Source: CAD feature listing. Evaluate the final solid. Frame: model axes, mm. A direction names the side the tool comes from. Give positions to 0.01 mm unless a question says otherwise; leave off trailing zeros. Order: outer loops, then holes, each group sorted by start corner. A loop starts at its lowest first (then second) coordinate and runs counter-clockwise, first axis right, second up. Notation, with made-up numbers: (84, 9) -> (100, 9) arc R22 cw to (100, 16) -> close; hole circle Ø1 at (87, -12.75). An arc over 180 degrees is marked (long way). Use one line per item in the form item = value. Start each with the question number.
from build123d import *

# Parameters (mm, degrees)
BOSS_EXTRUDE1_DEPTH = 80
SKETCH3_W           = 20
SKETCH3_H           = 40
CUT_EXTRUDE1_DEPTH  = 25
SKETCH4_W           = 55
SKETCH4_H           = 5
CUT_EXTRUDE2_DEPTH  = 40
SKETCH6_W           = 20
SKETCH6_H           = 5
CUT_EXTRUDE3_DEPTH  = 40
SKETCH7_W           = 20
SKETCH7_H           = 10
CUT_EXTRUDE4_DEPTH  = 20
SKETCH8_W           = 10
SKETCH8_H           = 10
BOSS_EXTRUDE2_DEPTH = 20
SKETCH9_W           = 15
SKETCH9_H           = 10
CUT_EXTRUDE5_DEPTH  = 20
SKETCH11_W          = 15
SKETCH11_H          = 5
CUT_EXTRUDE6_DEPTH  = 40


with BuildPart() as part:
    # Sketch1 → Boss-Extrude1 (new body)
    with BuildSketch(Plane(origin=(0, 0, 0), x_dir=(0, 0, -1), z_dir=(1, 0, 0))):
        Polygon((0, 0), (0, -15), (40, -15), (40, 25), (0, 25), (0, 10), (20, 10), (20, 0), align=None)
    extrude(amount=-BOSS_EXTRUDE1_DEPTH)

    # Sketch3 → Cut-Extrude1 (cut)
    with BuildSketch(Plane.XZ.offset(15)):
        with Locations((-40, -20)):
            Rectangle(SKETCH3_W, SKETCH3_H)
    extrude(amount=-CUT_EXTRUDE1_DEPTH, mode=Mode.SUBTRACT)

    # Sketch4 → Cut-Extrude2 (cut)
    with BuildSketch(Plane.XY):
        with Locations((-37.5, 12.5)):
            Rectangle(SKETCH4_W, SKETCH4_H)
    extrude(amount=-CUT_EXTRUDE2_DEPTH, mode=Mode.SUBTRACT)

    # Sketch6 → Cut-Extrude3 (cut)
    with BuildSketch(Plane.XY):
        with Locations((-20, -2.5)):
            Rectangle(SKETCH6_W, SKETCH6_H)
    extrude(amount=-CUT_EXTRUDE3_DEPTH, mode=Mode.SUBTRACT)

    # Sketch7 → Cut-Extrude4 (cut)
    with BuildSketch(Plane.XY.offset(-20)):
        with Locations((-20, 5)):
            Rectangle(SKETCH7_W, SKETCH7_H)
    extrude(amount=-CUT_EXTRUDE4_DEPTH, mode=Mode.SUBTRACT)

    # Sketch8 → Boss-Extrude2 (add)
    with BuildSketch(Plane.XY.offset(-20)):
        with Locations((-5, 5)):
            Rectangle(SKETCH8_W, SKETCH8_H)
    extrude(amount=BOSS_EXTRUDE2_DEPTH)

    # Sketch9 → Cut-Extrude5 (cut)
    with BuildSketch(Plane.XY.offset(-20)):
        with Locations((-57.5, 5)):
            Rectangle(SKETCH9_W, SKETCH9_H)
    extrude(amount=-CUT_EXTRUDE5_DEPTH, mode=Mode.SUBTRACT)

    # Sketch11 → Cut-Extrude6 (cut)
    with BuildSketch(Plane(origin=(0, 0, -40), x_dir=(-1, 0, 0), z_dir=(0, 0, -1))):
        with Locations((57.5, -2.5)):
            Rectangle(SKETCH11_W, SKETCH11_H)
    extrude(amount=-CUT_EXTRUDE6_DEPTH, mode=Mode.SUBTRACT)


solid = part.part
1) Cut plane C-C, the plane x = -53.5. Return the cut outline in (y, z), plus the area to 3 significant figures.
2) Cut plane B-B, the plane y = -4. Return the cut outline in (x, z).
3) Draft query along Y for faces 1 (the face through (-50, -10, -20)), 2 (the face through (-15, -15, -20)), 3 (the face through (-73, 0, -10)), 4 (the face through (-38, 15, -20)). Return one class per face: +Y half, -Y half, draft (parallel to the pull), parting line (faces both ways), or undercut.
4) Reachability of faces 5 (the face through (-80, 5, -24)), 6 (the face through (-72, 10, -10)), 7 (the face through (-20, -5, -20)), 8 (the face through (-30, -10, -20)) from +Z, -Z, +X, -X, +Y, -Y: full face, straight path, thin tool, end or side. Return the list, or none.
5) Cut plane D-D, the plane z = -27. Return the cut outline in (x, y).
6) Cut plane A-A, the plane z = -5. Return the cut outline in (x, y), plus the area to 3 significant figures.
7) Material intervals for probe 1 along X at (y, z) = (4.5, -25); probe 2 along Y at (x, z) = (-24.5, -2.5); probe 3 along X at (y, z) = (-12.5, -30.5), sorted ascending.
8) Pin query (flat end, axial travel): pin 1 (3 mm diameter, centred on x = -37.5, z = -20.5, fed in from -Y); pin 2 (5 mm diameter, centred on x = -71, y = 6.5, fed in from +Z). Return the tip coordinate at first contact, or that it passes through.
Output values:
q1.outline = (-15, -40) -> (-5, -40) -> (-5, 0) -> (-15, 0) -> close; (15, -40) -> (25, -40) -> (25, 0) -> (15, 0) -> close
q1.area = 800 mm^2
q2.outline = (-80, -40) -> (-65, -40) -> (-65, 0) -> (-80, 0) -> close; (-10, -40) -> (0, -40) -> (0, 0) -> (-10, 0) -> close
q3.face_1 = draft
q3.face_2 = -Y half
q3.face_3 = undercut
q3.face_4 = undercut
q4.face_5 = +Z, -Z, -X, +Y, -Y
q4.face_6 = +Z, -X
q4.face_7 = +Z, -Z
q4.face_8 = +Z, -Z, -Y
q5.outline = (-80, -15) -> (-50, -15) -> (-50, -5) -> (-65, -5) -> (-65, 15) -> (-10, 15) -> (-10, -5) -> (-30, -5) -> (-30, -15) -> (0, -15) -> (0, 25) -> (-80, 25) -> close
q6.outline = (-80, -15) -> (-50, -15) -> (-50, -5) -> (-65, -5) -> (-65, 0) -> (-80, 0) -> close; (-80, 10) -> (-65, 10) -> (-65, 15) -> (-10, 15) -> (-10, -5) -> (-30, -5) -> (-30, -15) -> (0, -15) -> (0, 25) -> (-80, 25) -> close
q6.area = 1,750 mm^2
q7.probe_1 = -80 to -65, -10 to 0
q7.probe_2 = -15 to -5, 15 to 25
q7.probe_3 = -80 to -50, -30 to 0
q8.pin_1 = 15
q8.pin_2 = -20
